from build123d import *

# Parameters (mm, degrees)
F0_W     = 387
F0_H     = 630
F1_DEPTH = 120.5
F3_W     = 177
F3_H     = 323
F5_DEPTH = 145.5
F2_W     = 323
F2_H     = 566
F6_DEPTH = 193
F4_W     = 177
F4_H     = 566
F7_DEPTH = 211
F8_W     = 177
F8_H     = 323
F9_DEPTH = 315.001


with BuildPart() as f1:
    # F0 (on Right) → F1 (new body, symmetric)
    with BuildSketch(Plane.YZ):
        Rectangle(F0_W, F0_H)
    extrude(amount=F1_DEPTH, both=True)


with BuildPart() as f5:
    # F3 (on Top) → F5 (new body, symmetric)
    with BuildSketch(Plane.XY):
        Rectangle(F3_W, F3_H)
    extrude(amount=F5_DEPTH, both=True)


with BuildPart() as f6_tool:
    # F2 (on face) → F6 (new body)
    with BuildSketch(Plane.YZ.offset(120.5)):
        Rectangle(F2_W, F2_H)
    extrude(amount=-F6_DEPTH)


with BuildPart() as f1_1:
    add(f1.part)

    # F6: cut by f6_tool
    add(f6_tool.part, mode=Mode.SUBTRACT)


with BuildPart() as f5_1:
    add(f5.part)

    # F6: cut by f6_tool
    add(f6_tool.part, mode=Mode.SUBTRACT)


with BuildPart() as f7_tool:
    # F4 (on Front) → F7 (new body, symmetric)
    with BuildSketch(Plane.XZ):
        Rectangle(F4_W, F4_H)
    extrude(amount=F7_DEPTH, both=True)


with BuildPart() as f1_2:
    add(f1_1.part)

    # F7: cut by f7_tool
    add(f7_tool.part, mode=Mode.SUBTRACT)

    # F8 (on Top) → F9 (cut, through all)
    with BuildSketch(Plane.XY):
        Rectangle(F8_W, F8_H)
    extrude(amount=F9_DEPTH, mode=Mode.SUBTRACT)


with BuildPart() as f5_2:
    add(f5_1.part)

    # F7: cut by f7_tool
    add(f7_tool.part, mode=Mode.SUBTRACT)


solid = f1_2.part
The model under review builds one solid part; all positions refer to its coordinate system, in mm. A direction names the side the tool comes from. Round coordinates to 2 decimals unless told otherwise and drop trailing zeros. Loops run counter-clockwise (first coordinate to the right, second up) from the corner with the lowest first, then second, coordinate; pieces in that order, holes last. Notation, with made-up numbers: (-37.5, 64) -> (1.5, 64) arc R25 ccw to (1.5, 82) -> close; hole circle Ø8 at (-12.75, 66). An arc over 180 degrees is marked (long way). Return JSON: item names as keys, results as strings.
(1) Add section C-C on z = -80. Write out the cut boundary in (x, y).
Solved:
{"outline": "(-120.5, -193.5) -> (-88.5, -193.5) -> (-88.5, 193.5) -> (-120.5, 193.5) -> close; (88.5, -193.5) -> (120.5, -193.5) -> (120.5, -161.5) -> (88.5, -161.5) -> close; (88.5, 161.5) -> (120.5, 161.5) -> (120.5, 193.5) -> (88.5, 193.5) -> close"}
(2) Add section A-A on x = -20.5. Write out the cut boundary in (y, z).
Solved:
{"outline": "(-193.5, -315) -> (193.5, -315) -> (193.5, -283) -> (-193.5, -283) -> close; (-193.5, 283) -> (-161.5, 283) -> (-161.5, 315) -> (-193.5, 315) -> close; (161.5, 283) -> (193.5, 283) -> (193.5, 315) -> (161.5, 315) -> close"}
(3) For pin 1 (8 mm diameter, centred on x = -48.5, y = -81.5, fed in from +Z); pin 2 (2 mm diameter, centred on y = 60.5, z = 33, fed in from +X), all flat-tipped, find the tip position at first contact; note any pin that passes through.
Solved:
{"pin 1": "z = -283", "pin 2": "x = -88.5"}
(4) Add section D-D on x = 98. Write out the cut boundary in (y, z).
Solved:
{"outline": "(-193.5, -315) -> (193.5, -315) -> (193.5, 315) -> (-193.5, 315) -> close; hole (-161.5, -283) -> (161.5, -283) -> (161.5, 283) -> (-161.5, 283) -> close"}
(5) For faces 1 (the flat face through (104, -2, 283)), 2 (the flat face through (88.5, -2, 299)), 3 (the flat face through (-1, 177, 283)), list the 3-axis set-ups (+Z, -Z, +X, -X, +Y, -Y) from which the entire face can be reached by the end or side of a thin tool; tool diameter is ignored.
Solved:
{"face 1": "+X", "face 2": "+Z", "face 3": "+Y, -Y"}
(6) Add section B-B on y = 154.5. Write out the cut boundary in (x, z).
Solved:
{"outline": "(-120.5, -315) -> (120.5, -315) -> (120.5, -283) -> (-88.5, -283) -> (-88.5, 315) -> (-120.5, 315) -> close; (88.5, 283) -> (120.5, 283) -> (120.5, 315) -> (88.5, 315) -> close"}
(7) For line 1 (Y direction, x = 109.5, z = 84); line 2 (Z direction, x = 54.5, y = -171); line 3 (X direction, y = -168.5, z = -212.5), list the stretches that pass through material, from the lowest coordinate up.
Solved:
{"line 1": "-193.5 to -161.5, 161.5 to 193.5", "line 2": "-315 to -283, 283 to 315", "line 3": "-120.5 to -88.5, 88.5 to 120.5"}
(8) The part is to be moulded in two halves that separate along Z. For faces 4 (the flat face through (105, -161.5, -4)), 5 (the flat face through (2, -3, -315)), 6 (the flat face through (90, -193.5, -1)), 7 (the flat face through (-105, -3, 315)), say which applies: released by +Z, released by -Z, zero draft, split by the parting line, or undercut.
Solved:
{"face 4": "undercut", "face 5": "released by -Z", "face 6": "zero draft", "face 7": "released by +Z"}
